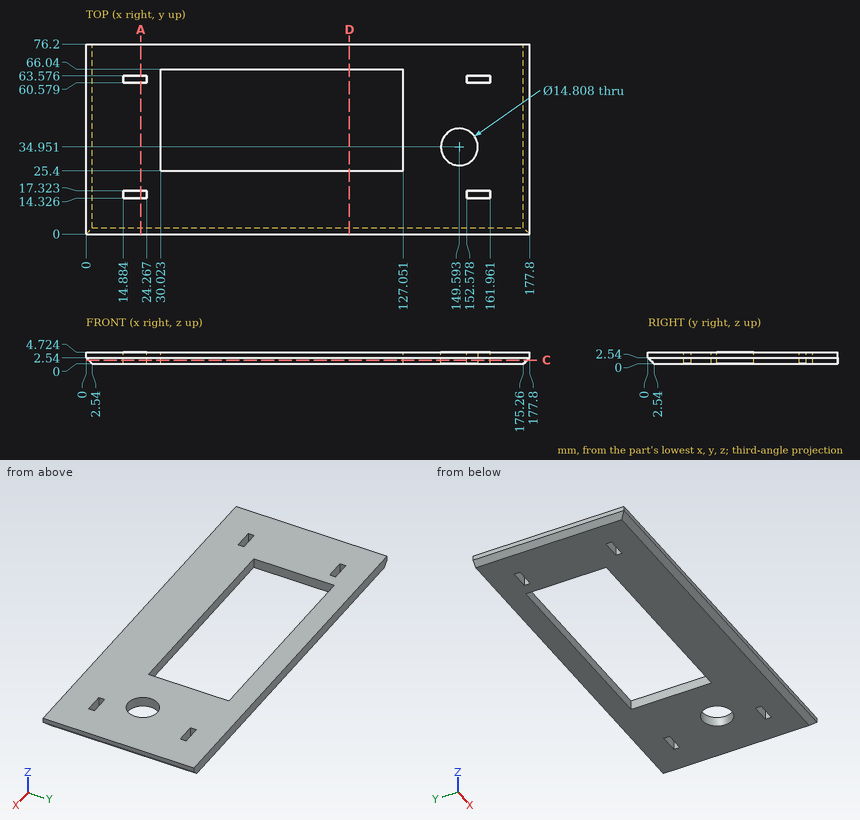
Check sheet for the drawn part. Datum: minimum x, y, z corner. Units: mm. Round coordinates to 2 decimals unless told otherwise and drop trailing zeros. Order: outer loops, then holes, each group sorted by start corner. A loop starts at its lowest first (then second) coordinate and runs counter-clockwise, first axis right, second up. Notation, with made-up numbers: (13, 41) - (30, 41) arc R16 cw to (30, 59) - close; hole circle Ø7 at (88, 53.5). An arc over 180 degrees is marked (long way). Use a Markdown table: item, result. Add a question column.
(1) Depth check by flat-ended pin: pin 1 (1.4 mm diameter, centred on x = 21.5, z = 2.5, fed in from -Y); pin 2 (1.5 mm diameter, centred on x = 57.5, y = 27, fed in from -Z); pin 3 (0.9 mm diameter, centred on y = 16, z = 2, fed in from -X). Enter the tip coordinate at first touch or a pass-through.
(2) Material ranges on line 1 along X through (y, z) = (51, 3.1); line 2 along Y through (x, z) = (89, 3.2); line 3 along Y through (x, z) = (109.5, 1.25), recorded low to high. Write a range as [from, to].
(3) Sectioned sample at A-A, the plane x = 22. Enter the section's corners in (y, z) (1 decimal).
(4) Sectioned sample at C-C, the plane z = 1.55. Count the separate pieces of the cut face and the enclosed holes in it.
(5) Sectioned sample at D-D, the plane x = 105.5. Enter the section's corners in (y, z) (1 decimal).
Answers below:
| question | item | result |
|---|---|---|
| 1 | pin 1 | y = 0 |
| 1 | pin 2 | through |
| 1 | pin 3 | x = 0.09 |
| 2 | line 1 | [0, 30.02], [127.05, 177.8] |
| 2 | line 2 | [0, 25.4], [66.04, 76.2] |
| 2 | line 3 | [1.29, 25.4], [66.04, 76.2] |
| 3 | outline | (0, 2.5) - (2.5, 0) - (14.3, 0) - (14.3, 4.7) - (0, 4.7) - close; (17.3, 0) - (60.6, 0) - (60.6, 4.7) - (17.3, 4.7) - close; (63.6, 0) - (76.2, 0) - (76.2, 4.7) - (63.6, 4.7) - close |
| 4 | separate pieces | 1 |
| 4 | enclosed holes | 6 |
| 5 | outline | (0, 2.5) - (2.5, 0) - (25.4, 0) - (25.4, 4.7) - (0, 4.7) - close; (66, 0) - (76.2, 0) - (76.2, 4.7) - (66, 4.7) - close |
